Source: CAD feature listing. Evaluate the final solid. Frame: model axes, mm. A direction names the side the tool comes from. Coordinates: 2 decimals unless noted, no trailing zeros. Order: outer loops, then holes, each group sorted by start corner. A loop starts at its lowest first (then second) coordinate and runs counter-clockwise, first axis right, second up.
```python
from build123d import *

# Parameters (mm, degrees)
SKETCH1_W           = 6.096
SKETCH1_H           = 7.62
BOSS_EXTRUDE1_DEPTH = 3.048


with BuildPart() as part:
    # Sketch1 → Boss-Extrude1 (new, symmetric)
    with BuildSketch(Plane(origin=(0, 0, 0), x_dir=(1, 0, 0), z_dir=(0, 1, 0))):
        with BuildLine():
            Line((-49.53, 45.72), (-10.668, 45.72))
            Line((-10.668, 45.72), (-10.668, 38.1))
            Line((-10.668, 38.1), (-4.572, 38.1))
            Line((-4.572, 38.1), (-4.572, 45.72))
            Line((-4.572, 45.72), (4.572, 45.72))
            Line((4.572, 45.72), (4.572, 38.1))
            Line((4.572, 38.1), (10.668, 38.1))
            Line((10.668, 38.1), (10.668, 45.72))
            Line((10.668, 45.72), (49.53, 45.72))
            Line((49.53, 45.72), (49.53, 38.1))
            Line((49.53, 38.1), (55.626, 38.1))
            Line((55.626, 38.1), (55.626, 27.94))
            Line((55.626, 27.94), (49.53, 27.94))
            Line((49.53, 27.94), (49.53, 1.208143374))
            Line((49.53, 1.208143374), (55.626, 1.208143374))
            Line((55.626, 1.208143374), (55.626, -8.951856626))
            Line((55.626, -8.951856626), (49.53, -8.951856626))
            Line((49.53, -8.951856626), (49.53, -16.571856626))
            Line((49.53, -16.571856626), (55.626, -16.571856626))
            Line((55.626, -16.571856626), (55.626, -29.271856626))
            Line((55.626, -29.271856626), (21.019827136, -42.136821893))
            ThreePointArc((21.019827136, -42.136821893), (17.95098831, -44.911778638), (17.631953735, -49.036869377))
            Line((17.631953735, -49.036869377), (25.187729856, -73.287029113))
            ThreePointArc((25.187729856, -73.287029113), (26.234780075, -75.207903536), (27.939063878, -76.579577488))
            ThreePointArc((27.939063878, -76.579577488), (41.468907088, -82.632484358), (55.626, -87.022365809))
            Line((55.626, -87.022365809), (55.626, -132.617292876))
            Line((55.626, -132.617292876), (10.668, -132.617292876))
            Line((10.668, -132.617292876), (10.668, -122.457292876))
            Line((10.668, -122.457292876), (4.572, -122.457292876))
            Line((4.572, -122.457292876), (4.572, -94.642365809))
            Line((4.572, -94.642365809), (10.668, -94.642365809))
            Line((10.668, -94.642365809), (10.668, -87.022365809))
            Line((10.668, -87.022365809), (4.572, -87.022365809))
            Line((4.572, -87.022365809), (4.572, -80.672365809))
            Line((4.572, -80.672365809), (-4.572, -80.672365809))
            Line((-4.572, -80.672365809), (-4.572, -87.022365809))
            Line((-4.572, -87.022365809), (-10.668, -87.022365809))
            Line((-10.668, -87.022365809), (-10.668, -94.642365809))
            Line((-10.668, -94.642365809), (-4.572, -94.642365809))
            Line((-4.572, -94.642365809), (-4.572, -122.457292876))
            Line((-4.572, -122.457292876), (-10.668, -122.457292876))
            Line((-10.668, -122.457292876), (-10.668, -132.617292876))
            Line((-10.668, -132.617292876), (-49.53, -132.617292876))
            Line((-49.53, -132.617292876), (-49.53, -124.997292876))
            Line((-49.53, -124.997292876), (-55.626, -124.997292876))
            Line((-55.626, -124.997292876), (-55.626, -116.107292876))
            Line((-55.626, -116.107292876), (-49.53, -116.107292876))
            Line((-49.53, -116.107292876), (-49.53, -105.947292876))
            Line((-49.53, -105.947292876), (-55.626, -105.947292876))
            Line((-55.626, -105.947292876), (-55.626, -97.057292876))
            Line((-55.626, -97.057292876), (-49.53, -97.057292876))
            Line((-49.53, -97.057292876), (-49.53, -85.359826344))
            ThreePointArc((-49.53, -85.359826344), (-38.527111219, -81.479756652), (-27.939063878, -76.579577488))
            ThreePointArc((-27.939063878, -76.579577488), (-26.234780075, -75.207903536), (-25.187729856, -73.287029113))
            Line((-25.187729856, -73.287029113), (-17.631953735, -49.036869377))
            ThreePointArc((-17.631953735, -49.036869377), (-17.95098831, -44.911778638), (-21.019827136, -42.136821893))
            Line((-21.019827136, -42.136821893), (-55.626, -29.271856626))
            Line((-55.626, -29.271856626), (-55.626, -16.571856626))
            Line((-55.626, -16.571856626), (-49.53, -16.571856626))
            Line((-49.53, -16.571856626), (-49.53, -8.951856626))
            Line((-49.53, -8.951856626), (-55.626, -8.951856626))
            Line((-55.626, -8.951856626), (-55.626, 1.208143374))
            Line((-55.626, 1.208143374), (-49.53, 1.208143374))
            Line((-49.53, 1.208143374), (-49.53, 27.94))
            Line((-49.53, 27.94), (-55.626, 27.94))
            Line((-55.626, 27.94), (-55.626, 38.1))
            Line((-55.626, 38.1), (-49.53, 38.1))
            Line((-49.53, 38.1), (-49.53, 45.72))
        make_face()
        with Locations((7.62, -25.461856626)):
            Rectangle(SKETCH1_W, SKETCH1_H, mode=Mode.SUBTRACT)
        with Locations((-7.62, -25.461856626)):
            Rectangle(SKETCH1_W, SKETCH1_H, mode=Mode.SUBTRACT)
    extrude(amount=BOSS_EXTRUDE1_DEPTH, both=True)


solid = part.part
```
1. Section query D-D on z = -7. Return loops of the section in (x, y).
Findings:
outline: (-49.53, -3.05) - (49.53, -3.05) - (49.53, 3.05) - (-49.53, 3.05) - close
2. Draft query along X for faces 1 (the face through (-4.572, 0, 26)), 2 (the face through (-49.53, 0, -42)), 3 (the face through (1, 3.048, 42)). Return one class per face: released by +X, released by -X, zero draft, split by the parting line, or undercut.
Findings:
face 1: undercut
face 2: released by -X
face 3: zero draft
3. Section query C-C on y = -1.75. Count the separate pieces of the cut face and the enclosed holes in it, plus the area to 3 significant figures.
Findings:
separate pieces: 1
enclosed holes: 2
area: 15,100 mm2
4. Access query for faces 4 (the face through (-4.572, 0, 108)), 5 (the face through (-8, 0, -38.1)), 6 (the face through (41.275, 0.043, 82.559)), 7 (the face through (8, 0, 87.022)), 8 (the face through (-53, 0, -1.208)). Directions: +Z, -Z, +X, -X, +Y, -Y. A direction counts if a zero-diameter tool reaches every point of the face in a straight line with its end or side. Return the directions, or none.
Findings:
face 4: +Z, +Y, -Y
face 5: -Z, +Y, -Y
face 6: +X, +Y, -Y
face 7: +Y, -Y
face 8: -X, +Y, -Y
5. Ray query, line 1 (Z direction, x = 9.5, y = 2.5); line 2 (X direction, y = 1.75, z = 112.5); line 3 (X direction, y = 2.75, z = 123.5). Return the intervals inside material, ascending.
Findings:
line 1: z = -38.1 to 21.65, 29.27 to 87.02, 94.64 to 122.46
line 2: x = -49.53 to -4.57, 4.57 to 55.63
line 3: x = -55.63 to -10.67, 10.67 to 55.63
6. Section query B-B on x = 30. Return loops of the section in (y, z), plus the area to 3 significant figures.
Findings:
outline: (-3.05, -45.72) - (3.05, -45.72) - (3.05, 38.8) - (-3.05, 38.8) - close; (-3.05, 77.63) - (3.05, 77.63) - (3.05, 132.62) - (-3.05, 132.62) - close
area: 850 mm2
7. Section query A-A on z = 26. Return loops of the section in (x, y), plus the area to 3 significant figures.
Findings:
outline: (-55.63, -3.05) - (-10.67, -3.05) - (-10.67, 3.05) - (-55.63, 3.05) - close; (-4.57, -3.05) - (4.57, -3.05) - (4.57, 3.05) - (-4.57, 3.05) - close; (10.67, -3.05) - (55.63, -3.05) - (55.63, 3.05) - (10.67, 3.05) - close
area: 604 mm2
8. Pin query (flat end, axial travel): P1, Ø2, axis at y = -2, z = 90, coming from the -X side; P2, Ø1.8, axis at x = -52.5, y = 0, coming from the +Z side; P3, Ø1.8, axis at x = -52.5, y = -1, coming from the -Z side. Return the tip coordinate at first contact, or that it passes through.
Findings:
P1: stops at x = -49.53
P2: stops at z = 125
P3: stops at z = -38.1
